Source: CAD feature listing. Evaluate the final solid. Frame: model axes, mm. A direction names the side the tool comes from. Round coordinates to 2 decimals unless told otherwise and drop trailing zeros. Order: outer loops, then holes, each group sorted by start corner. A loop starts at its lowest first (then second) coordinate and runs counter-clockwise, first axis right, second up. Notation, with made-up numbers: M 63.25,38.5 L 113.25,38.5 A14 cw 113.25,42.5 Z; hole C 25,-24.75 d9. An arc over 180 degrees is marked long. Answer in a Markdown table with one row per item. Add a question column.
```python
from build123d import *

# Parameters (mm, degrees)
BOSS_EXTRUDE3_DEPTH              = 14.5
SKETCH8_R                        = 6.884606738
CUT_EXTRUDE3_DEPTH               = 88
CUT_EXTRUDE4_DEPTH               = 2.4
CUT_EXTRUDE5_DEPTH               = 2.4
F_39_0_11811024_DIAMETER_HOLE1_D = 3.000000096


with BuildPart() as part:
    # Sketch6 → Boss-Extrude3 (new body)
    with BuildSketch(Plane(origin=(0, 0, 0), x_dir=(1, 0, 0), z_dir=(0, 1, 0))):
        Polygon((-16.836914056, 5.783353512), (13.163085944, 5.783353512), (33.163085944, -49.166194877), (-36.836914056, -49.166194877), align=None)
    extrude(amount=BOSS_EXTRUDE3_DEPTH)

    # Sketch8 → Cut-Extrude3 (cut)
    with BuildSketch(Plane.XY.offset(49.166194877)):
        with Locations((-1.836914056, 0)):
            Circle(SKETCH8_R)
    extrude(amount=-CUT_EXTRUDE3_DEPTH, mode=Mode.SUBTRACT)

    # Sketch9 → Cut-Extrude4 (cut)
    with BuildSketch(Plane(origin=(0, 14.5, 0), x_dir=(1, 0, 0), z_dir=(0, 1, 0))):
        Polygon((-21.661914056, -27.308299801), (-18.911914056, -25.72058656), (-18.911914056, -22.54516008), (-21.661914056, -20.95744684), (-24.411914056, -22.54516008), (-24.411914056, -25.72058656), align=None)
        Polygon((-26.486914056, -46.224526633), (-23.736914056, -44.636813392), (-23.736914056, -41.461386912), (-26.486914056, -39.873673672), (-29.236914056, -41.461386912), (-29.236914056, -44.636813392), align=None)
        Polygon((22.813085944, -46.224526633), (25.563085944, -44.636813392), (25.563085944, -41.461386912), (22.813085944, -39.873673672), (20.063085944, -41.461386912), (20.063085944, -44.636813392), align=None)
        Polygon((18.031463076, -27.308299801), (20.781463076, -25.72058656), (20.781463076, -22.54516008), (18.031463076, -20.95744684), (15.281463076, -22.54516008), (15.281463076, -25.72058656), align=None)
        Polygon((-16.836914056, -8.392072969), (-14.086914056, -6.804359728), (-14.086914056, -3.628933248), (-16.836914056, -2.041220008), (-19.586914056, -3.628933248), (-19.586914056, -6.804359728), align=None)
        Polygon((13.163085944, -8.392072969), (15.913085944, -6.804359728), (15.913085944, -3.628933248), (13.163085944, -2.041220008), (10.413085944, -3.628933248), (10.413085944, -6.804359728), align=None)
    extrude(amount=-CUT_EXTRUDE4_DEPTH, mode=Mode.SUBTRACT)

    # Sketch10 → Cut-Extrude5 (cut)
    with BuildSketch(Plane.XZ):
        Polygon((-26.486914056, 39.873673672), (-23.736914056, 41.461386912), (-23.736914056, 44.636813392), (-26.486914056, 46.224526633), (-29.236914056, 44.636813392), (-29.236914056, 41.461386912), align=None)
        Polygon((-21.661914056, 20.95744684), (-18.911914056, 22.54516008), (-18.911914056, 25.72058656), (-21.661914056, 27.308299801), (-24.411914056, 25.72058656), (-24.411914056, 22.54516008), align=None)
        Polygon((18.031463076, 20.95744684), (20.781463076, 22.54516008), (20.781463076, 25.72058656), (18.031463076, 27.308299801), (15.281463076, 25.72058656), (15.281463076, 22.54516008), align=None)
        Polygon((22.813085944, 39.873673672), (25.563085944, 41.461386912), (25.563085944, 44.636813392), (22.813085944, 46.224526633), (20.063085944, 44.636813392), (20.063085944, 41.461386912), align=None)
        Polygon((-16.836914056, 2.041220008), (-14.086914056, 3.628933248), (-14.086914056, 6.804359728), (-16.836914056, 8.392072969), (-19.586914056, 6.804359728), (-19.586914056, 3.628933248), align=None)
        Polygon((13.163085944, 2.041220008), (15.913085944, 3.628933248), (15.913085944, 6.804359728), (13.163085944, 8.392072969), (10.413085944, 6.804359728), (10.413085944, 3.628933248), align=None)
    extrude(amount=-CUT_EXTRUDE5_DEPTH, mode=Mode.SUBTRACT)

    # #39 (0.11811024) Diameter Hole1 (through all)
    with Locations(Plane(origin=(-16.836914056, 14.5, 5.216646488), x_dir=(0, 0, 1), z_dir=(0, 1, 0))):
        with Locations((0, 0), (0, 30), (18.916226832, 34.868377132), (18.916226832, -4.825), (37.832453664, -9.65), (37.832453664, 39.65)):
            Hole(F_39_0_11811024_DIAMETER_HOLE1_D / 2)


solid = part.part
```
(1) Access query for faces 1 (the face through (-27.4, 7.18, 44.24)), 2 (the face through (-20.27, 13.32, 21.76)), 3 (the face through (-23.056, 1.183, 21.762)). Directions: +Z, -Z, +X, -X, +Y, -Y. A direction counts if a zero-diameter tool reaches every point of the face in a straight line with its end or side. Return the directions, or none.
(2) Line query: line 1 (X direction, y = 10.5, z = 25); line 2 (X direction, y = 1, z = 22.5); line 3 (X direction, y = 10, z = 4). Output: solid intervals per line, ascending. Write a range as from..to.
(3) Draft query along X for faces 4 (the face through (-2, 9, -5.783)), 5 (the face through (-25.13, 13.32, 45.44)). Return one class per face: +X half, -X half, draft (parallel to the pull), parting line (faces both ways), or undercut.
(4) Pin query (flat end, axial travel): pin 1 (1.6 mm diameter, centred on x = -27, z = 42, fed in from +Y); pin 2 (3 mm diameter, centred on y = 3, z = 38.5, fed in from +X); pin 3 (0.7 mm diameter, centred on y = 13.5, z = 25, fed in from +X); pin 4 (2.5 mm diameter, centred on x = -21.66, z = 24.13, fed in from +Y). Return the tip coordinate at first contact, or that it passes through.
(5) Cut plane A-A (y = 4.5). Return loops of the section in (x, z).
(6) Cut plane C-C (z = 43). Count the separate pieces of the cut face and the enclosed holes in it, and give its area (3 significant figures).
(7) Cut plane B-B (y = 11). Return loops of the section in (x, z), and give its area (3 significant figures).
Answer list:
| question | item | result |
|---|---|---|
| 1 | face 1 | +Y, -Y |
| 1 | face 2 | +Y |
| 1 | face 3 | -Y |
| 2 | line 1 | -28.04..-22.89, -20.44..16.81, 19.26..24.37 |
| 2 | line 2 | -27.13..-24.33, -18.99..-8.65, 4.97..15.36, 20.7..23.46 |
| 2 | line 3 | -20.4..-17.71, -15.96..12.29, 14.04..16.72 |
| 3 | face 4 | draft |
| 3 | face 5 | undercut |
| 4 | pin 1 | y = 12.1 |
| 4 | pin 2 | x = 29.83 |
| 4 | pin 3 | x = 24.49 |
| 4 | pin 4 | through |
| 5 | outline | M -36.84,49.17 L -16.84,-5.78 L -7.05,-5.78 L -7.05,49.17 Z; M 3.37,-5.78 L 13.16,-5.78 L 33.16,49.17 L 3.37,49.17 Z; hole C -26.49,43.05 d3; hole C -21.66,24.13 d3; hole C -16.84,5.22 d3; hole C 13.16,5.22 d3; hole C 18.03,24.13 d3; hole C 22.81,43.05 d3 |
| 6 | separate pieces | 3 |
| 6 | enclosed holes | 0 |
| 6 | area | 764 mm² |
| 7 | outline | M -36.84,49.17 L -16.84,-5.78 L 13.16,-5.78 L 33.16,49.17 Z; hole C -26.49,43.05 d3; hole C -21.66,24.13 d3; hole C -16.84,5.22 d3; hole C 13.16,5.22 d3; hole C 18.03,24.13 d3; hole C 22.81,43.05 d3 |
| 7 | area | 2,710 mm² |
